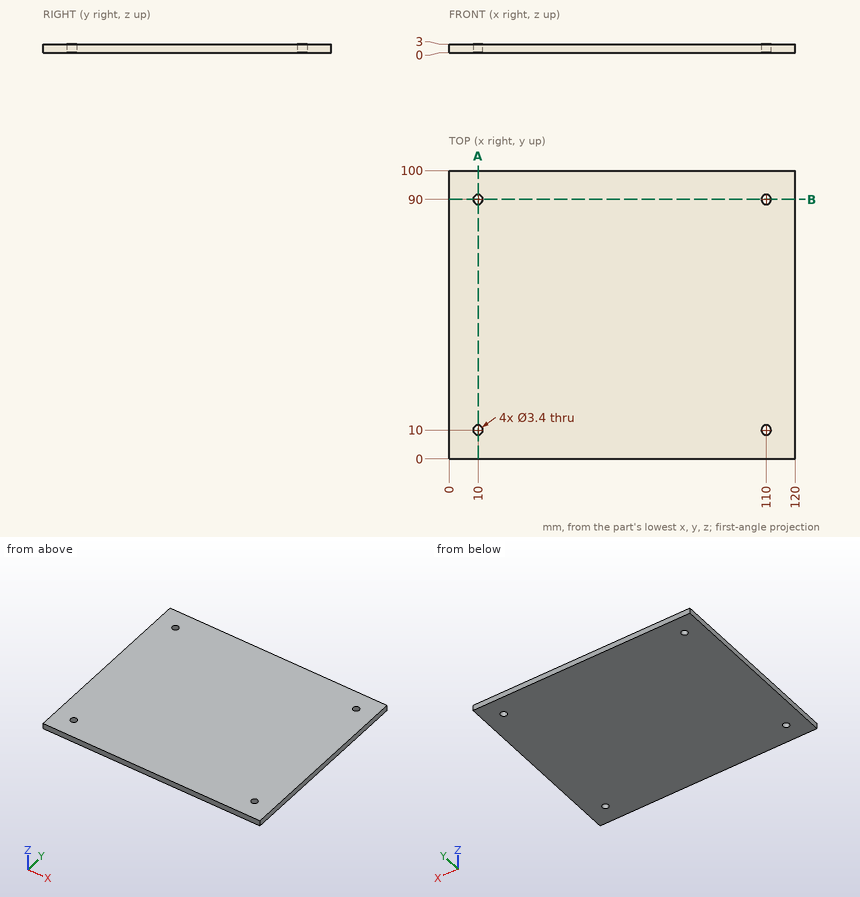
Drawing for the job (mm, zero at the part's lowest x, y, z). Round coordinates to 2 decimals unless told otherwise and drop trailing zeros. Order: outer loops, then holes, each group sorted by start corner. A loop starts at its lowest first (then second) coordinate and runs counter-clockwise, first axis right, second up. Notation, with made-up numbers: M 36,-22 L 88,-22 A25 ccw 88,6 Z; hole C 18.5,-2 d9. An arc over 180 degrees is marked long. Use one line per item in the form item = value.
Q1. Probe L1, parallel to X at y = 90, z = 1.85; L2, parallel to Y at x = 10, z = 1.1; L3, parallel to Y at x = 10.5, z = 1.5. List the from-to ranges inside material, lowest first.
Recorded:
L1 = 0 to 8.3, 11.7 to 108.3, 111.7 to 120
L2 = 0 to 8.3, 11.7 to 88.3, 91.7 to 100
L3 = 0 to 8.38, 11.62 to 88.38, 91.62 to 100
Q2. Flat gauge pin, fed straight in: P1, Ø2, axis at x = 110, y = 10, coming from the -Z side. Where does the tip first touch, or does it go through?
Recorded:
P1 = through
Q3. Saw through at A-A on x = 10. Give the cut face in (y, z), then the cut area to 3 significant figures.
Recorded:
outline = M 0,0 L 8.3,0 L 8.3,3 L 0,3 Z; M 11.7,0 L 88.3,0 L 88.3,3 L 11.7,3 Z; M 91.7,0 L 100,0 L 100,3 L 91.7,3 Z
area = 280 mm^2
Q4. Saw through at B-B on y = 90. Give the cut face in (x, z), then the cut area to 3 significant figures.
Recorded:
outline = M 0,0 L 8.3,0 L 8.3,3 L 0,3 Z; M 11.7,0 L 108.3,0 L 108.3,3 L 11.7,3 Z; M 111.7,0 L 120,0 L 120,3 L 111.7,3 Z
area = 340 mm^2
